```python
from build123d import *

# Parameters (mm, degrees)
F0_R     = 23.8125
F1_DEPTH = 9.525
F2_R     = 15.875
F3_DEPTH = 15.875
F4_R     = 12.7
F5_DEPTH = 25.4
F6_R     = 10.3251
F7_DEPTH = 50.801
F8_SIZE  = 1.524
F9_SIZE  = 0.762


with BuildPart() as f1:
    # F0 (on Front) → F1 (new body)
    with BuildSketch(Plane.XZ):
        Circle(F0_R)
    extrude(amount=F1_DEPTH)

    # F2 (on face) → F3 (join)
    with BuildSketch(Plane.XZ.offset(9.525)):
        Circle(F2_R)
    extrude(amount=F3_DEPTH)

    # F4 (on face) → F5 (join)
    with BuildSketch(Plane.XZ.offset(25.4)):
        Circle(F4_R)
    extrude(amount=F5_DEPTH)

    # F6 (on face) → F7 (cut, through all)
    with BuildSketch(Plane.XZ.offset(50.8)):
        Circle(F6_R)
    extrude(amount=-F7_DEPTH, mode=Mode.SUBTRACT)

    # F8
    f8_edges = [f1.edges().sort_by_distance(p)[0] for p in [
        (-15.875, -25.4, 0),
    ]]
    chamfer(f8_edges, length=F8_SIZE)

    # F9
    f9_edges = [f1.edges().sort_by_distance(p)[0] for p in [
        (-23.8125, -9.525, 0),
        (-23.8125, 0, 0),
        (-10.3251, 0, 0),
    ]]
    chamfer(f9_edges, length=F9_SIZE)


solid = f1.part
```
CAD build for the part. Positions are in the model's coordinates, mm. A direction names the side the tool comes from. Give positions to 0.01 mm unless a question says otherwise; leave off trailing zeros. Order: outer loops, then holes, each group sorted by start corner. A loop starts at its lowest first (then second) coordinate and runs counter-clockwise, first axis right, second up. Notation, with made-up numbers: M 89.25,-29 L 116.25,-29 A20 ccw 116.25,-20 Z; hole C 39.5,-20.75 d2. An arc over 180 degrees is marked long. Put each result on its own line as item: value. Start each with the question number.
(1) Flat gauge pins, fed straight in: pin 1 Ø5 at (y, z) = (-15, 8.5) entering from +X; pin 2 Ø5 at (x, y) = (10.5, -8.5) entering from +Z; pin 3 Ø4 at (x, y) = (-16, -32) entering from +Z; pin 4 Ø5 at (y, z) = (-30, -0.5) entering from -X. Where does each tip first touch, or does it go through?
(2) Which spindle directions (+Z, -Z, +X, -X, +Y, -Y) get a long thin tool onto all of the face, cutting with end or side? Do faces 1 (the flat face through (-1.9, -50.8, 10.4)), 2 (the flat face through (1, -25.4, -13)). Say none if no direction does.
(3) Saw through at A-A, the plane z = 0. Write the cut outline in (x, y) (1 decimal).
(4) Mould opens along Z. For faces 3 (the cylindrical face through (9.54, -26.13, -3.95)), 4 (the cylindrical face through (-18.897, -4.706, -14.49)), 5 (the flat face through (9.9, 0, 5.4)) say: +Z half, -Z half, draft (parallel to the pull), parting line (faces both ways), or undercut.
(5) Saw through at D-D, the plane y = -39. Write the cut outline in (x, z), then the cut area to 3 significant figures.
(6) Drill centre lines: line 1 along Z through (x, y) = (0, -22) (3 decimals); line 2 along Z through (x, y) = (0, -28); line 3 along Y through (x, z) = (5, 19) (3 decimals). Where is each one in solid material? Low to high.
(7) Saw through at B-B, the plane x = 0. Write the cut outline in (y, z) (1 decimal).
(8) Saw through at C-C, the plane y = -20.5. Write the cut outline in (x, z) (3 decimals).
Check result:
1. pin 1: stops at x = 14.7
1. pin 2: stops at z = 22.43
1. pin 3: passes through
1. pin 4: stops at x = -12.7
2. face 1: +Z, -Z, +X, -X, -Y
2. face 2: -Y
3. outline: M -23.8,-8.8 L -23.1,-9.5 L -15.9,-9.5 L -15.9,-23.9 L -14.4,-25.4 L -12.7,-25.4 L -12.7,-50.8 L -10.3,-50.8 L -10.3,-0.8 L -11.1,0 L -23.1,0 L -23.8,-0.8 Z; M 10.3,-50.8 L 12.7,-50.8 L 12.7,-25.4 L 14.4,-25.4 L 15.9,-23.9 L 15.9,-9.5 L 23.1,-9.5 L 23.8,-8.8 L 23.8,-0.8 L 23.1,0 L 11.1,0 L 10.3,-0.8 Z
4. face 3: undercut
4. face 4: parting line
4. face 5: draft
5. outline: C 0,0 d25.4; hole C 0,0 d20.65
5. area: 172 mm2
6. line 1: z = -15.875 to -10.325, 10.325 to 15.875
6. line 2: z = -12.7 to -10.33, 10.33 to 12.7
6. line 3: y = -9.525 to 0
7. outline: M -50.8,-12.7 L -25.4,-12.7 L -25.4,-14.4 L -23.9,-15.9 L -9.5,-15.9 L -9.5,-23.1 L -8.8,-23.8 L -0.8,-23.8 L 0,-23.1 L 0,-11.1 L -0.8,-10.3 L -50.8,-10.3 Z; M -50.8,10.3 L -0.8,10.3 L 0,11.1 L 0,23.1 L -0.8,23.8 L -8.8,23.8 L -9.5,23.1 L -9.5,15.9 L -23.9,15.9 L -25.4,14.4 L -25.4,12.7 L -50.8,12.7 Z
8. outline: C 0,0 d31.75; hole C 0,0 d20.65
